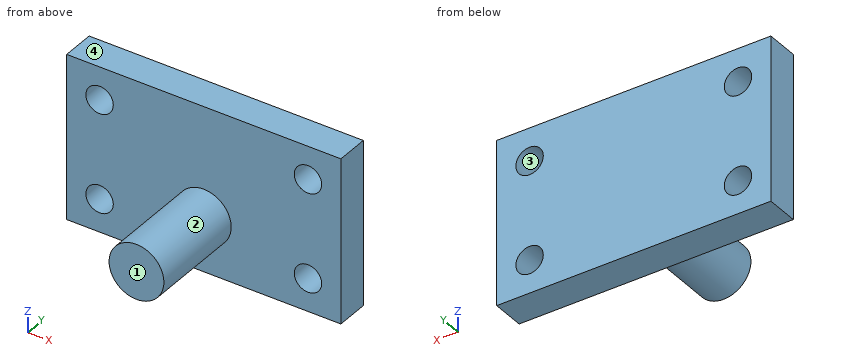
```python
from build123d import *

# Parameters (mm, degrees)
SKETCH2_W           = 250
SKETCH2_H           = 150
BOSS_EXTRUDE1_DEPTH = 15
SKETCH3_R           = 12.5
CUT_EXTRUDE1_DEPTH  = 149.828760661
SKETCH4_R           = 25
BOSS_EXTRUDE2_DEPTH = 90


with BuildPart() as part:
    # Sketch2 → Boss-Extrude1 (new, symmetric)
    with BuildSketch(Plane(origin=(0, 0, 0), x_dir=(1, 0, 0), z_dir=(0, 1, 0))):
        Rectangle(SKETCH2_W, SKETCH2_H)
    extrude(amount=BOSS_EXTRUDE1_DEPTH, both=True)

    # Sketch3 → Cut-Extrude1 (cut, through all)
    with BuildSketch(Plane(origin=(0, 15, 0), x_dir=(1, 0, 0), z_dir=(0, 1, 0))):
        with Locations(Location((-95, -45, 0), (0, 0, 270))):
            Circle(SKETCH3_R)
        with Locations(Location((-95, 45, 0), (0, 0, 270))):
            Circle(SKETCH3_R)
        with Locations(Location((95, -45, 0), (0, 0, 90))):
            Circle(SKETCH3_R)
        with Locations(Location((95, 45, 0), (0, 0, 90))):
            Circle(SKETCH3_R)
    extrude(amount=-CUT_EXTRUDE1_DEPTH, mode=Mode.SUBTRACT)

    # Sketch4 → Boss-Extrude2 (add)
    with BuildSketch(Plane.XZ.offset(15)):
        with Locations(Location((0, -25, 0), (0, 0, 90))):
            Circle(SKETCH4_R)
    extrude(amount=BOSS_EXTRUDE2_DEPTH)


solid = part.part
```
Build history of the part. All positions in model axes, mm. Face numbers are marked on the shaded views. Round coordinates to 2 decimals unless told otherwise and drop trailing zeros. Write each loop counter-clockwise with the first axis right and the second up, starting at its lowest first coordinate (ties: lowest second). Pieces come first, ordered by that corner, then holes. Notation, with made-up numbers: (-9, 72.25) - (14, 72.25) arc R37 cw to (14, 111.25) - close; hole circle Ø4 at (14, -24.75). An arc over 180 degrees is marked (long way). Answer as CSV lines item,"result".
Q1. Cut at B-B (x = 95). Write the cut outline in (y, z).
Report:
outline,"(-15, -75) - (15, -75) - (15, -57.5) - (-15, -57.5) - close; (-15, -32.5) - (15, -32.5) - (15, 32.5) - (-15, 32.5) - close; (-15, 57.5) - (15, 57.5) - (15, 75) - (-15, 75) - close"
Q2. Drop flat-ended pins along their axis: pin 1 (4 mm diameter, centred on x = 34.5, z = 22.5, fed in from -Y); pin 2 (1.5 mm diameter, centred on x = -1, y = -81.5, fed in from -Z); pin 3 (2 mm diameter, centred on y = -54.5, z = -36, fed in from +X). Give the stop position or say it passes through.
Report:
pin 1,"stops at y = -15"
pin 2,"stops at z = -50"
pin 3,"stops at x = 22.91"
Q3. Cut at C-C (y = 6.5). Write the cut outline in (x, z).
Report:
outline,"(-125, -75) - (125, -75) - (125, 75) - (-125, 75) - close; hole circle Ø25 at (-95, -45); hole circle Ø25 at (-95, 45); hole circle Ø25 at (95, -45); hole circle Ø25 at (95, 45)"
Q4. Cut at A-A (z = -45). Write the cut outline in (x, y), and give its area (3 significant figures).
Report:
outline,"(-125, -15) - (-107.5, -15) - (-107.5, 15) - (-125, 15) - close; (-82.5, -15) - (-15, -15) - (-15, -105) - (15, -105) - (15, -15) - (82.5, -15) - (82.5, 15) - (-82.5, 15) - close; (107.5, -15) - (125, -15) - (125, 15) - (107.5, 15) - close"
area,"8,700 mm^2"
Q5. Drill centre lines: probe 1 along X at (y, z) = (-7.5, -45); probe 2 along Z at (x, y) = (95, 1.75); probe 3 along Y at (x, z) = (34, 27). Where is each one in solid material? Low to high. Write a range as [from, to].
Report:
probe 1,"x = [-125, -107.5], [-82.5, 82.5], [107.5, 125]"
probe 2,"z = [-75, -57.5], [-32.5, 32.5], [57.5, 75]"
probe 3,"y = [-15, 15]"
Q6. Cut at D-D (x = 0). Write the cut outline in (y, z).
Report:
outline,"(-105, -50) - (-15, -50) - (-15, -75) - (15, -75) - (15, 75) - (-15, 75) - (-15, 0) - (-105, 0) - close"
Q7. Pull direction Z, two halves, no side cores. Call the marked faces 1, 2, 3 and 4: +Z half, -Z half, draft (parallel to the pull), parting line (faces both ways), or undercut.
Report:
face 1,"draft"
face 2,"parting line"
face 3,"undercut"
face 4,"+Z half"
